```python
from build123d import *

# Parameters (mm, degrees)
ESQUISSE1_W      = 80
ESQUISSE1_H      = 80
ESQUISSE1_R      = 2.5
ESQUISSE1_R_2    = 1.5
ESQUISSE1_R_3    = 2
EXTRUSION1_DEPTH = 3
CONG_1_R         = 2


with BuildPart() as part:
    # Esquisse1 → Extrusion1 (new body)
    with BuildSketch(Plane(origin=(0, 0, 0), x_dir=(1, 0, 0), z_dir=(0, 1, 0))):
        with Locations((40, 40)):
            Rectangle(ESQUISSE1_W, ESQUISSE1_H)
        with Locations((40, 40)):
            Circle(ESQUISSE1_R, mode=Mode.SUBTRACT)
        with Locations((60, 40)):
            Circle(ESQUISSE1_R, mode=Mode.SUBTRACT)
        with Locations((57.67766953, 57.67766953)):
            Circle(ESQUISSE1_R_2, mode=Mode.SUBTRACT)
        with Locations((22.32233047, 22.32233047)):
            Circle(ESQUISSE1_R_2, mode=Mode.SUBTRACT)
        with Locations((22.32233047, 57.67766953)):
            Circle(ESQUISSE1_R_2, mode=Mode.SUBTRACT)
        with Locations((57.67766953, 22.32233047)):
            Circle(ESQUISSE1_R_2, mode=Mode.SUBTRACT)
        with Locations((6, 74)):
            Circle(ESQUISSE1_R_3, mode=Mode.SUBTRACT)
        with Locations((74, 74)):
            Circle(ESQUISSE1_R_3, mode=Mode.SUBTRACT)
        with Locations((74, 6)):
            Circle(ESQUISSE1_R_3, mode=Mode.SUBTRACT)
        with Locations((6, 6)):
            Circle(ESQUISSE1_R_3, mode=Mode.SUBTRACT)
        with BuildLine():
            Line((19, 44), (29, 44))
            ThreePointArc((29, 44), (31.828427125, 42.828427125), (33, 40))
            ThreePointArc((33, 40), (31.828427125, 37.171572875), (29, 36))
            Line((29, 36), (19, 36))
            ThreePointArc((19, 36), (16.171572875, 37.171572875), (15, 40))
            ThreePointArc((15, 40), (16.171572875, 42.828427125), (19, 44))
        make_face(mode=Mode.SUBTRACT)
    extrude(amount=EXTRUSION1_DEPTH)

    # Congé1
    cong_1_edges = [part.edges().sort_by_distance(p)[0] for p in [
        (0, 1.5, -80),
        (80, 1.5, -80),
        (80, 1.5, 0),
        (0, 1.5, 0),
    ]]
    fillet(cong_1_edges, radius=CONG_1_R)


solid = part.part
```
CAD build for the part. Positions are in the model's coordinates, mm. A direction names the side the tool comes from. Round coordinates to 2 decimals unless told otherwise and drop trailing zeros. Write each loop counter-clockwise with the first axis right and the second up, starting at its lowest first coordinate (ties: lowest second). Pieces come first, ordered by that corner, then holes. Notation, with made-up numbers: (-19.5, 40.25) - (25.5, 40.25) arc R23 ccw to (25.5, 65.25) - close; hole circle Ø9 at (55.5, -9.5). An arc over 180 degrees is marked (long way). Return JSON: item names as keys, results as strings. Group by question number.
Item 1: Mould opens along Z. For faces 3 (the face through (0.57, 1.52, -0.6)), 4 (the face through (24, 1, -36)), 5 (the face through (39, 0, -49)) say: +Z half, -Z half, draft (parallel to the pull), parting line (faces both ways), or undercut.
Item 2: Band-saw the part on A-A on x = 74. List the corners of the cut face in (y, z).
Item 3: Band-saw the part on B-B on z = -74. List the corners of the cut face in (x, y), plus the area to 3 significant figures.
Item 4: Band-saw the part on C-C on x = 40. List the corners of the cut face in (y, z), plus the area to 3 significant figures.
Item 5: 3-axis set-ups, long thin cutter, end or side, ignore diameter. For faces 1 (the face through (24, 1, -44)), 2 (the face through (39, 3, -49)): which of +Z, -Z, +X, -X, +Y, -Y reach the whole face in a straight line?
Item 6: Probe probe 1 along Z at (x, y) = (6, 1); probe 2 along X at (y, z) = (2.15, -40); probe 3 along X at (y, z) = (2.3, -6). List the from-to ranges inside material, lowest first.
Resolved:
{
 "1": {"face 3": "+Z half", "face 4": "undercut", "face 5": "draft"},
 "2": {"outline": "(0, -80) - (3, -80) - (3, -76) - (0, -76) - close; (0, -72) - (3, -72) - (3, -8) - (0, -8) - close; (0, -4) - (3, -4) - (3, 0) - (0, 0) - close"},
 "3": {"outline": "(0, 0) - (4, 0) - (4, 3) - (0, 3) - close; (8, 0) - (72, 0) - (72, 3) - (8, 3) - close; (76, 0) - (80, 0) - (80, 3) - (76, 3) - close", "area": "216 mm²"},
 "4": {"outline": "(0, -80) - (3, -80) - (3, -42.5) - (0, -42.5) - close; (0, -37.5) - (3, -37.5) - (3, 0) - (0, 0) - close", "area": "225 mm²"},
 "5": {"face 1": "+Y, -Y", "face 2": "+Z, -Z, +X, -X, +Y"},
 "6": {"probe 1": "z = -80 to -76, -72 to -8, -4 to 0", "probe 2": "x = 0 to 15, 33 to 37.5, 42.5 to 57.5, 62.5 to 80", "probe 3": "x = 0 to 4, 8 to 72, 76 to 80"}
}
